Model file for the job. Use its own axes, mm. Face numbers are marked on the shaded views. A direction names the side the tool comes from. Coordinates: 2 decimals unless noted, no trailing zeros. Write each loop counter-clockwise with the first axis right and the second up, starting at its lowest first coordinate (ties: lowest second). Pieces come first, ordered by that corner, then holes.
Q1. Band-saw the part on C-C, the plane z = 28. Write the cut outline in (x, y).
Q2. Band-saw the part on D-D, the plane y = -34. Write the cut outline in (x, z).
Q3. Pull direction Z, two halves, no side cores. Call the marked faces 4, 5, 6 and 7: released by +Z, released by -Z, zero draft, split by the parting line, or undercut.
Q4. Drill centre lines: probe 1 along Z at (x, y) = (9.5, -47); probe 2 along Z at (x, y) = (22, -44); probe 3 along Z at (x, y) = (64.5, -19). Where is each one in solid material? Low to high.
Q5. Band-saw the part on A-A, the plane y = -47.5. Write the cut outline in (x, z).
Q6. Pin check, flat tips, straight feed: P1, Ø5, axis at x = 22.5, z = 7, coming from the +Y side; P2, Ø1.8, axis at y = -29, z = 4.5, coming from the -X side; P3, Ø8, axis at x = 41.5, y = -43.5, coming from the -Z side. Stop position of each tip, or through.
Q7. Band-saw the part on B-B, the plane x = 41. Write the cut outline in (y, z), plus the area to 3 significant figures.
Q8. Which spindle directions (+Z, -Z, +X, -X, +Y, -Y) get a long thin tool onto all of the face, cutting with end or side? Do the marked faces 1, 2 and 3. Say none if no direction does.
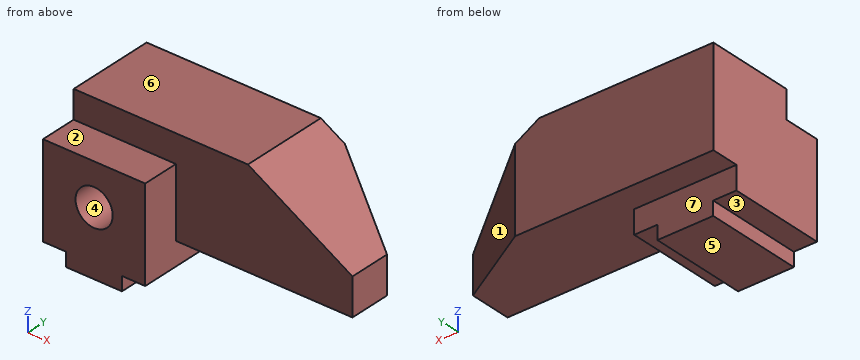
from build123d import *

# Parameters (mm, degrees)
F0_W      = 120
F0_H      = 58
F1_DEPTH  = 54
F2_W      = 10
F2_H      = 6
F3_DEPTH  = 54.001
F5_DEPTH  = 16
F6_R      = 8
F7_DEPTH  = 22
F8_W      = 44
F8_H      = 16
F9_DEPTH  = 12
F11_DEPTH = 58.001


with BuildPart() as f1:
    # F0 (on Front) → F1 (new body)
    with BuildSketch(Plane.XZ):
        with Locations((60, 29)):
            Rectangle(F0_W, F0_H)
    extrude(amount=F1_DEPTH)

    # F2 (on face) → F3 (cut, through all)
    with BuildSketch(Plane.XZ.offset(54)):
        Polygon((34, 6), (34, 0), (120, 0), (120, 16), (44, 16), (44, 6), align=None)
        Polygon((120, 58), (75, 58), (120, 32.019238), align=None)
        with Locations((5, 3)):
            Rectangle(F2_W, F2_H)
    extrude(amount=-F3_DEPTH, mode=Mode.SUBTRACT)

    # F4 (on face) → F5 (cut)
    with BuildSketch(Plane.XZ.offset(54)):
        Polygon((75, 58), (0, 58), (0, 46), (44, 46), (44, 16), (120, 16), (120, 32.019238), align=None)
    extrude(amount=-F5_DEPTH, mode=Mode.SUBTRACT)

    # F6 (on face) → F7 (cut)
    with BuildSketch(Plane.XZ.offset(54)):
        with Locations((22, 28)):
            Circle(F6_R)
    extrude(amount=-F7_DEPTH, mode=Mode.SUBTRACT)

    # F8 (on face) → F9 (cut)
    with BuildSketch(Plane(origin=(0, 0, 0), x_dir=(-1, 0, 0), z_dir=(0, 1, 0))):
        with Locations((-22, 8)):
            Rectangle(F8_W, F8_H)
    extrude(amount=-F9_DEPTH, mode=Mode.SUBTRACT)

    # F10 (on face) → F11 (cut, through all)
    with BuildSketch(Plane.XY.offset(58)):
        Polygon((85.358984, 0), (120, -20), (120, 0), align=None)
    extrude(amount=-F11_DEPTH, mode=Mode.SUBTRACT)


solid = f1.part
Answer sheet:
1. outline: (0, -54) - (14, -54) - (14, -32) - (30, -32) - (30, -54) - (44, -54) - (44, -38) - (120, -38) - (120, -20) - (85.36, 0) - (0, 0) - close
2. outline: (0, 6) - (10, 6) - (10, 0) - (34, 0) - (34, 6) - (44, 6) - (44, 16) - (120, 16) - (120, 32.02) - (75, 58) - (0, 58) - close; hole circle Ø16 at (22, 28)
3. face 4: undercut
3. face 5: released by -Z
3. face 6: released by +Z
3. face 7: zero draft
4. probe 1: z = 6 to 46
4. probe 2: z = 0 to 20, 36 to 46
4. probe 3: z = 16 to 58
5. outline: (0, 6) - (10, 6) - (10, 0) - (34, 0) - (34, 6) - (44, 6) - (44, 46) - (0, 46) - close; hole circle Ø16 at (22, 28)
6. P1: stops at y = -12
6. P2: stops at x = 10
6. P3: stops at z = 6
7. outline: (-54, 6) - (-12, 6) - (-12, 16) - (0, 16) - (0, 58) - (-38, 58) - (-38, 46) - (-54, 46) - close
7. area: 2,500 mm2
8. face 1: +Z, -Z, +X, +Y
8. face 2: +Z, +X, -X, -Y
8. face 3: -Z, -X, +Y, -Y
